```python
from build123d import *

# Parameters (mm, degrees)
F0_W     = 304.8
F0_H     = 254
F1_DEPTH = 63.5
F2_R     = 31.75
F3_R     = 31.74999


# Not quite as in the source:
# - a fillet or chamfer is up to 0.001 mm smaller than in the source, because OpenCascade refuses the exact size


with BuildPart() as f1:
    # F0 (on Top) → F1 (new body)
    with BuildSketch(Plane.XY):
        Rectangle(F0_W, F0_H)
    extrude(amount=F1_DEPTH)

    # F2
    f2_edges = [f1.edges().sort_by_distance(p)[0] for p in [
        (152.4, 0, 63.5),
        (0, 127, 63.5),
        (-152.4, 0, 63.5),
        (0, -127, 63.5),
    ]]
    fillet(f2_edges, radius=F2_R)

    # F3 (radius 31.75 in the source; OpenCascade refuses exactly that, so slightly less here)
    f3_edges = [f1.edges().sort_by_distance(p)[0] for p in [
        (152.4, 0, 0),
        (0, 127, 0),
        (-152.4, 0, 0),
        (0, -127, 0),
    ]]
    fillet(f3_edges, radius=F3_R)


solid = f1.part
```
The listing builds one solid part. Answer for the finished solid, in the listing's coordinates (mm). Give positions to 0.01 mm unless a question says otherwise; leave off trailing zeros. Loops run counter-clockwise (first coordinate to the right, second up) from the corner with the lowest first, then second, coordinate; pieces in that order, holes last. Notation, with made-up numbers: (71, 82.5) - (128, 82.5) arc R13 ccw to (128, 98.5) - close; hole circle Ø5 at (-5, 12.25). An arc over 180 degrees is marked (long way). Return JSON: item names as keys, results as strings. Group by question number.
1. Find section D-D (z = 11.5). Write down the section's boundary in (x, y).
2. Straight lines are drawn through the part: line 1 (Y direction, x = -7, z = 33.5); line 2 (X direction, y = -20.5, z = 34); line 3 (Z direction, x = 132, y = -106.5). For each, find the intervals that lie inside material, in ascending order. Write a range as [from, to].
3. Given pin 1 Ø1.5 at (x, z) = (79.5, 11) entering from -Y; pin 2 Ø5 at (y, z) = (88, 17.5) entering from +X; pin 3 Ø3 at (y, z) = (-86, 37.5) entering from -X, each flat-ended and moving along its own axis, determine where each tip first touches the part or whether it passes through.
4. Find section C-C (z = 51). Write down the section's boundary in (x, y), then the cut area to 3 significant figures.
Verdict:
{
 "1": {"outline": "(-145.1, -119.7) - (145.1, -119.7) - (145.1, 119.7) - (-145.1, 119.7) - close"},
 "2": {"line 1": "y = [-126.95, 126.95]", "line 2": "x = [-152.32, 152.32]", "line 3": "z = [2.1, 61.4]"},
 "3": {"pin 1": "stops at y = -119.91", "pin 2": "stops at x = 150.15", "pin 3": "stops at x = -152.11"},
 "4": {"outline": "(-145.9, -120.5) - (145.9, -120.5) - (145.9, 120.5) - (-145.9, 120.5) - close", "area": "70,300 mm^2"}
}
